Work out the finished part from the listing and answer in its coordinate system (mm). Coordinates: 2 decimals unless noted, no trailing zeros. Order: outer loops, then holes, each group sorted by start corner. A loop starts at its lowest first (then second) coordinate and runs counter-clockwise, first axis right, second up. Notation, with made-up numbers: (51, 77) -> (76, 77) arc R19 cw to (76, 92) -> close; hole circle Ø6 at (55.25, -25.5). An arc over 180 degrees is marked (long way). Use one line per item in the form item = value.
Autodesk Inventor part; units mm, degrees
ref_plane "YZ Plane" through (0, 0, 0) normal (1, 0, 0) x (0, 1, 0)
ref_plane "XZ Plane" through (0, 0, 0) normal (0, 1, 0) x (-1, 0, 0)
ref_plane "XY Plane" through (0, 0, 0) normal (0, 0, 1) x (1, 0, 0)
sketch "Szkic1" plane through (0, 0, 0) normal (1, 0, 0) x (0, 1, 0)
  line L0 (-5.5, 10) -> (5.5, 10)
  line L1 (5.5, 10) -> (5.5, -10)
  line L2 (5.5, -10) -> (-5.5, -10)
  line L3 (-5.5, -10) -> (-5.5, 10)
  line L4 (-5.5, 10) -> (5.5, -10) construction
  line L5 (5.5, 10) -> (-5.5, -10) construction
  point P0 (0, 0)
  dimension "d0" = 20
  dimension "d1" = 11
extrude "Wyciągnięcie proste1" add sketch "Szkic1" along normal blind 6.5
sketch "Szkic2" plane through (6.5, 0, 0) normal (1, 0, 0) x (0, 0, -1)
  line L0 (-9.9535, -3.5) -> (10, -3.5) construction
  line L1 (10, -5.5) -> (10, 5.5)
  line L2 (-10, -5.5) -> (10, -5.5)
  circle A0 centre (-5, -3.5) radius 1.25
  circle A1 centre (5, -3.5) radius 1.25
  line L3 (-10, 5.5) -> (-10, -5.5)
  point P0 (0, 0)
  dimension "d4" = 2
  dimension "d5" = 5
  dimension "d6" = 5
  dimension "d7" = 2.5
  dimension "d8" = 2.5
extrude "Wyciągnięcie proste2" cut sketch "Szkic2" against normal through all
properties part number "Stop_sw" material "Tworzywo sztuczne ABS"
(1) Section B-B on z = -5 is taken. Write down the section's boundary in (x, y).
Data:
outline = (0, -5.5) -> (6.5, -5.5) -> (6.5, -4.75) -> (0, -4.75) -> close; (0, -2.25) -> (6.5, -2.25) -> (6.5, 5.5) -> (0, 5.5) -> close
(2) This flat-tipped pin is pushed along its axis until it touches: P1, Ø1.5, axis at y = -3.5, z = 5, coming from the +X side. Where does it stop, or does it pass through?
Data:
P1 = through
(3) Section A-A on y = -3.5 is taken. Write down the section's boundary in (x, z), plus the area to 3 significant figures.
Data:
outline = (0, -10) -> (6.5, -10) -> (6.5, -6.25) -> (0, -6.25) -> close; (0, -3.75) -> (6.5, -3.75) -> (6.5, 3.75) -> (0, 3.75) -> close; (0, 6.25) -> (6.5, 6.25) -> (6.5, 10) -> (0, 10) -> close
area = 97.5 mm²
(4) Straight lines are drawn through the part: line 1 along Y through (x, z) = (3, 5); line 2 along Z through (x, y) = (5.25, -2.5); line 3 along Z through (x, y) = (2, -3). For each, find the intervals that lie inside material, in ascending order.
Data:
line_1 = -5.5 to -4.75, -2.25 to 5.5
line_2 = -10 to -5.75, -4.25 to 4.25, 5.75 to 10
line_3 = -10 to -6.15, -3.85 to 3.85, 6.15 to 10
(5) Section C-C on x = 2.75 is taken. Write down the section's boundary in (y, z), plus the area to 3 significant figures.
Data:
outline = (-5.5, -10) -> (5.5, -10) -> (5.5, 10) -> (-5.5, 10) -> close; hole circle Ø2.5 at (-3.5, -5); hole circle Ø2.5 at (-3.5, 5)
area = 210 mm²
(6) The mould has two halves that part along Y. Classify faces 1 (the cylindrical face through (3.3, -3.45, 6.25)), 2 (the flat face through (3, 0, -10)), 3 (the flat face through (3, -5.5, 0)): released by +Y, released by -Y, zero draft, split by the parting line, or undercut.
Data:
face_1 = undercut
face_2 = zero draft
face_3 = released by -Y
